Part model, mm, in its own coordinate system. Face numbers are marked on the shaded views. A direction names the side the tool comes from. Give positions to 0.01 mm unless a question says otherwise; leave off trailing zeros. Write each loop counter-clockwise with the first axis right and the second up, starting at its lowest first coordinate (ties: lowest second). Pieces come first, ordered by that corner, then holes.
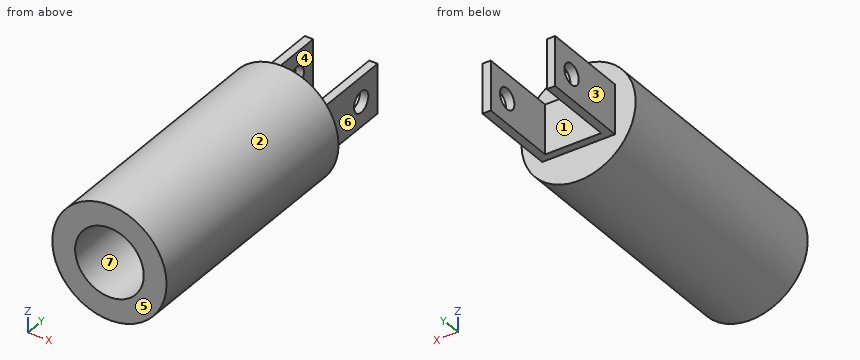
```python
from build123d import *

# Parameters (mm, degrees)
SKETCH1_W           = 4.826
SKETCH1_H           = 25.19045
BOSS_EXTRUDE1_DEPTH = 28.6258
SKETCH2_R           = 25.4
BOSS_EXTRUDE2_DEPTH = 145.034
SKETCH4_R           = 33.02
BOSS_EXTRUDE3_DEPTH = 145.034
SKETCH5_R           = 6.0325
CUT_EXTRUDE2_DEPTH  = 55.0512
SKETCH6_R           = 19.812
CUT_EXTRUDE3_DEPTH  = 106.934


with BuildPart() as part:
    # Sketch1 → Boss-Extrude1 (new body)
    with BuildSketch(Plane.XY):
        Polygon((37.2364, 24.806452693), (42.0624, 24.806452693), (42.0624, 50.3809), (37.2364, 50.3809), (37.2364, 25.19045), align=None)
        Polygon((21.0312, 4.572), (21.0312, 0), (42.0624, 0), (42.0624, 24.806452693), (37.2364, 24.806452693), (37.2364, 4.572), align=None)
        Polygon((0, 0), (21.0312, 0), (21.0312, 4.572), (4.826, 4.572), (4.826, 25.19045), (0, 25.19045), align=None)
        with Locations((2.413, 37.785675)):
            Rectangle(SKETCH1_W, SKETCH1_H)
    extrude(amount=BOSS_EXTRUDE1_DEPTH)

    # Sketch2 → Boss-Extrude2 (add)
    with BuildSketch(Plane.XZ):
        with Locations((21.0312, 14.3129)):
            Circle(SKETCH2_R)
    extrude(amount=BOSS_EXTRUDE2_DEPTH)

    # Sketch4 → Boss-Extrude3 (add)
    with BuildSketch(Plane(origin=(0, 0, 0), x_dir=(1, 0, 0), z_dir=(0, 1, 0))):
        with Locations((21.0312, -14.3129)):
            Circle(SKETCH4_R)
    extrude(amount=-BOSS_EXTRUDE3_DEPTH)

    # Sketch5 → Cut-Extrude2 (cut, through all)
    with BuildSketch(Plane(origin=(42.0624, 0, 0), x_dir=(0, 0, -1), z_dir=(1, 0, 0))):
        with Locations((-14.3129, 36.576)):
            Circle(SKETCH5_R)
    extrude(amount=-CUT_EXTRUDE2_DEPTH, mode=Mode.SUBTRACT)

    # Sketch6 → Cut-Extrude3 (cut)
    with BuildSketch(Plane.XZ.offset(145.034)):
        with Locations((21.0312, 14.3129)):
            Circle(SKETCH6_R)
    extrude(amount=-CUT_EXTRUDE3_DEPTH, mode=Mode.SUBTRACT)


solid = part.part
```
1) 3-axis set-ups, long thin cutter, end or side, ignore diameter. For the marked faces 4, 5, 6 and 7: which of +Z, -Z, +X, -X, +Y, -Y reach the whole face in a straight line?
Answers follow:
face 4: +Z, -Z, +Y
face 5: +Z, -Z, +X, -X, -Y
face 6: +Z, -Z, +X, +Y
face 7: -Y
2) Wall check: L1, parallel to X at y = 21, z = 25; L2, parallel to Z at x = 29, y = -109; L3, parallel to Z at x = 12.5, y = -102. Give the ranges that are in metal, low to high.
Answers follow:
L1: x = 0 to 4.83, 37.24 to 42.06
L2: z = -17.73 to -3.83, 32.45 to 46.36
L3: z = -17.59 to -3.57, 32.19 to 46.21
3) Saw through at C-C, the plane x = 15.5. Write the cut outline in (y, z).
Answers follow:
outline: (-145.03, -18.24) - (0, -18.24) - (0, 0) - (4.57, 0) - (4.57, 28.63) - (0, 28.63) - (0, 46.87) - (-145.03, 46.87) - (-145.03, 33.34) - (-38.1, 33.34) - (-38.1, -4.71) - (-145.03, -4.71) - close
4) Saw through at B-B, the plane z = 16.5. Write the cut outline in (x, y), then the cut area to 3 significant figures.
Answers follow:
outline: (-11.92, -145.03) - (1.34, -145.03) - (1.34, -38.1) - (40.72, -38.1) - (40.72, -145.03) - (53.98, -145.03) - (53.98, 0) - (42.06, 0) - (42.06, 30.95) - (37.24, 30.95) - (37.24, 4.57) - (4.83, 4.57) - (4.83, 30.95) - (0, 30.95) - (0, 0) - (-11.92, 0) - close; (0, 42.2) - (4.83, 42.2) - (4.83, 50.38) - (0, 50.38) - close; (37.24, 42.2) - (42.06, 42.2) - (42.06, 50.38) - (37.24, 50.38) - close
area: 5,870 mm2
5) Saw through at D-D, the plane z = 31. Write the cut outline in (x, y).
Answers follow:
outline: (-7.46, -145.03) - (10.35, -145.03) - (10.35, -38.1) - (31.71, -38.1) - (31.71, -145.03) - (49.52, -145.03) - (49.52, 0) - (-7.46, 0) - close
6) Saw through at A-A, the plane y = 18. Write the cut outline in (x, z), then the cut area to 3 significant figures.
Answers follow:
outline: (0, 0) - (4.83, 0) - (4.83, 28.63) - (0, 28.63) - close; (37.24, 0) - (42.06, 0) - (42.06, 28.63) - (37.24, 28.63) - close
area: 276 mm2
7) Two-plate mould, pull along X, no slides. Class the marked faces 1, 2 and 3: +X half, -X half, draft (parallel to the pull), parting line (faces both ways), or undercut.
Answers follow:
face 1: undercut
face 2: parting line
face 3: -X half
8) Pin check, flat tips, straight feed: pin 1 Ø4 at (x, z) = (15, 11.5) entering from -Y; pin 2 Ø21 at (x, y) = (15, 26.5) entering from -Z; pin 3 Ø14.5 at (y, z) = (32.5, 13) entering from +X. Stop position of each tip, or through.
Answers follow:
pin 1: stops at y = -38.1
pin 2: stops at z = 0
pin 3: stops at x = 42.06
